Can you work these out from the drawing? Everything is in mm from the part's minimum corner. A direction names the side the tool comes from. Round coordinates to 2 decimals unless told otherwise and drop trailing zeros. Order: outer loops, then holes, each group sorted by start corner. A loop starts at its lowest first (then second) coordinate and runs counter-clockwise, first axis right, second up. Notation, with made-up numbers: M 50,43 L 94,43 A28 cw 94,72 Z; hole C 43.5,-3 d7. An arc over 180 degrees is marked long. Answer as CSV lines item,"result". Start each with the question number.
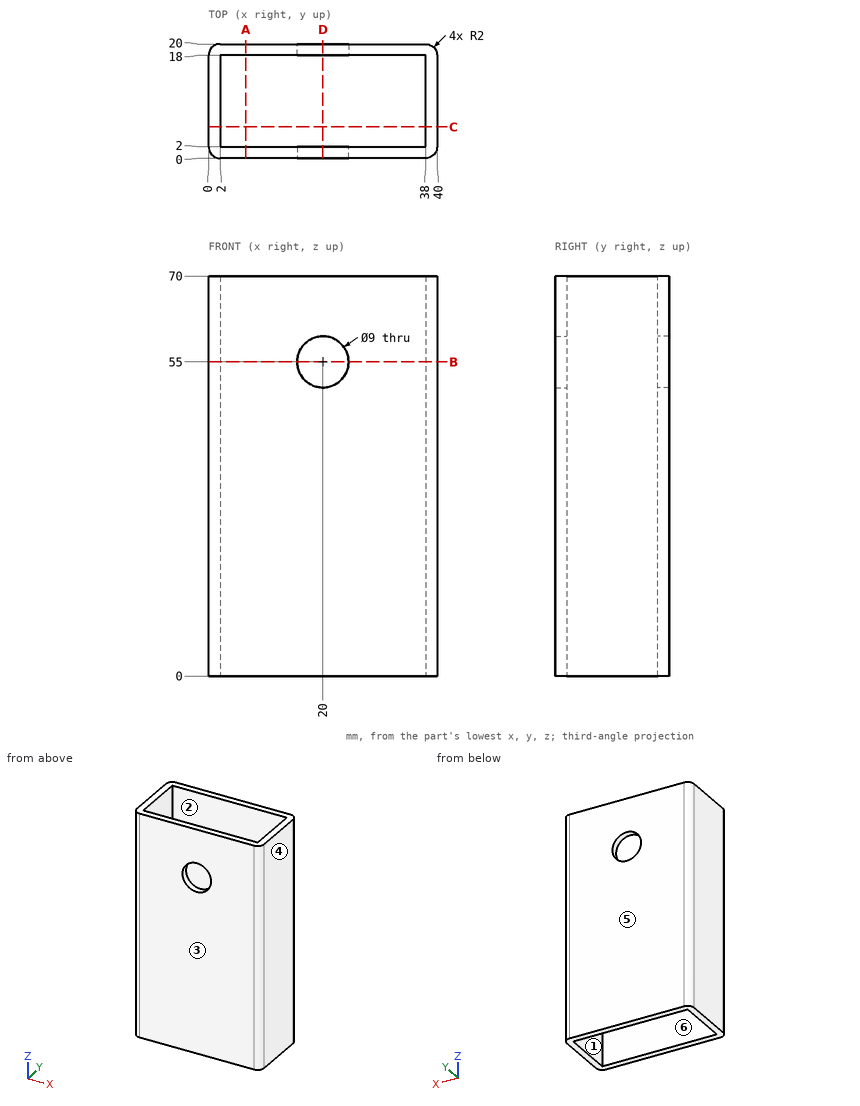
(1) I want a section at B-B on z = 55. Write out the boundary of the cut face in (x, y), and give its area (3 significant figures).
(2) I want a section at C-C on y = 5.5. Write out the boundary of the cut face in (x, z).
(3) I want a section at D-D on x = 20. Write out the boundary of the cut face in (y, z), and give its area (3 significant figures).
(4) I'm going to push flat-ended pins straight in: P1, Ø4, axis at x = 10.5, z = 61.5, coming from the -Y side; P2, Ø5, axis at x = 26, y = 5.5, coming from the -Z side. Where does each tip first touch, or does it pass through?
(5) For the marked faces 5 and 6, which set-ups out of +Z, -Z, +X, -X, +Y, -Y let a thin tool reach every point of the face, with its end or its side?
(6) If I drill on line 1 along Y through (x, z) = (21.5, 41.5); line 2 along X through (y, z) = (13, 45); line 3 along X through (y, z) = (19.65, 55), over which ranges is the centre line in solid material (lowest first)?
(7) If we mould it in two halves opening along X, with no side actions, what happens to the marked faces 1, 2, 3 and 4? For each: +X half, -X half, draft (parallel to the pull), parting line (faces both ways), or undercut.
(8) I want a section at A-A on x = 6.5. Write out the boundary of the cut face in (y, z), and give its area (3 significant figures).
From the geometry:
1,outline,"M 0,2 A2 ccw 2,0 L 15.5,0 L 15.5,2 L 2,2 L 2,18 L 15.5,18 L 15.5,20 L 2,20 A2 ccw 0,18 Z; M 24.5,0 L 38,0 A2 ccw 40,2 L 40,18 A2 ccw 38,20 L 24.5,20 L 24.5,18 L 38,18 L 38,2 L 24.5,2 Z"
1,area,"185 mm²"
2,outline,"M 0,0 L 2,0 L 2,70 L 0,70 Z; M 38,0 L 40,0 L 40,70 L 38,70 Z"
3,outline,"M 0,0 L 2,0 L 2,50.5 L 0,50.5 Z; M 0,59.5 L 2,59.5 L 2,70 L 0,70 Z; M 18,0 L 20,0 L 20,50.5 L 18,50.5 Z; M 18,59.5 L 20,59.5 L 20,70 L 18,70 Z"
3,area,"244 mm²"
4,P1,"y = 0"
4,P2,"through"
5,face 5,"+Z, -Z, +X, -X, +Y"
5,face 6,"+Z, -Z"
6,line 1,"0 to 2, 18 to 20"
6,line 2,"0 to 2, 38 to 40"
6,line 3,"0.87 to 15.5, 24.5 to 39.13"
7,face 1,"undercut"
7,face 2,"undercut"
7,face 3,"draft"
7,face 4,"+X half"
8,outline,"M 0,0 L 2,0 L 2,70 L 0,70 Z; M 18,0 L 20,0 L 20,70 L 18,70 Z"
8,area,"280 mm²"
